The figure shows three views and two pictorial views of one solid part (mm, origin at its lowest corner). Answer the questions. A direction names the side the tool comes from. Coordinates: 2 decimals unless noted, no trailing zeros. Order: outer loops, then holes, each group sorted by start corner. A loop starts at its lowest first (then second) coordinate and runs counter-clockwise, first axis right, second up. Notation, with made-up numbers: M -40,30 L -17,30 A28 cw -17,53 Z; hole C -13,-29.5 d3. An arc over 180 degrees is marked long. Write item = value, one per line. Start each with the question number.
Q1. Find section D-D on x = 19. Give the vertices of the cut face in (y, z).
Q2. Straight lines are drawn through the part: line 1 along Y through (x, z) = (149, 198); line 2 along Y through (x, z) = (54.5, 28); line 3 along Z through (x, y) = (148, 108). For each, find the intervals that lie inside material, in ascending order.
Q3. Find section A-A on z = 139. Give the vertices of the cut face in (x, y).
Q4. A tool of negligible diameter and unlimited length cuts with its end or side. For the marked faces 1 and 2, from which of +Z, -Z, +X, -X, +Y, -Y can it reach the whole face along a straight path? Write none if from no direction.
Q5. Each of these flat-tipped pins is pushed along its axis until it touches: P1, Ø1, axis at x = 135.5, y = 149.5, coming from the -Z side; P2, Ø2, axis at x = 86.5, y = 183, coming from the -Z side; P3, Ø4, axis at x = 142.5, z = 203, coming from the -Y side; P4, Ø6, axis at y = 71, z = 70.5, coming from the -X side. Where does it stop, or does it pass through?
Q6. Find section C-C on y = 107. Give the vertices of the cut face in (x, z).
Q7. Determine the mould class of the marked faces 3, 4 and 5 for opening direction Y: released by +Y, released by -Y, zero draft, split by the parting line, or undercut.
Q8. Find section B-B on x = 125. Give the vertices of the cut face in (y, z), and give its area (3 significant figures).
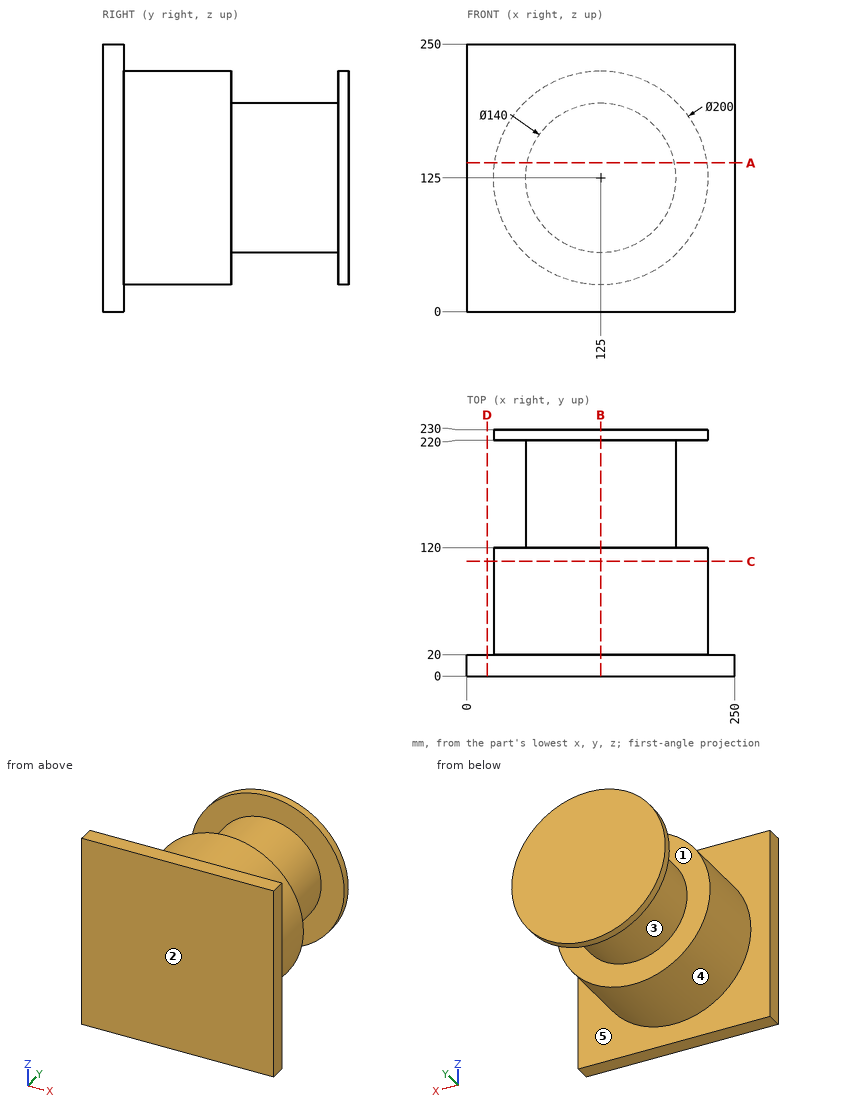
Findings below:
q1.outline = M 0,0 L 20,0 L 20,250 L 0,250 Z
q2.line_1 = 0 to 120, 220 to 230
q2.line_2 = 0 to 20
q2.line_3 = 27.68 to 222.32
q3.outline = M 0,0 L 250,0 L 250,20 L 224.02,20 L 224.02,120 L 193.59,120 L 193.59,220 L 224.02,220 L 224.02,230 L 25.98,230 L 25.98,220 L 56.41,220 L 56.41,120 L 25.98,120 L 25.98,20 L 0,20 Z
q4.face_1 = none
q4.face_2 = +Z, -Z, +X, -X, -Y
q5.P1 = 55.72
q5.P2 = 65.89
q5.P3 = 0
q5.P4 = 39.28
q6.outline = C 125,125 d200
q7.face_3 = undercut
q7.face_4 = zero draft
q7.face_5 = released by +Y
q8.outline = M 0,0 L 20,0 L 20,25 L 120,25 L 120,55 L 220,55 L 220,25 L 230,25 L 230,225 L 220,225 L 220,195 L 120,195 L 120,225 L 20,225 L 20,250 L 0,250 Z
q8.area = 41,000 mm^2
